```python
from build123d import *

# Parameters (mm, degrees)
BOSS_EXTRUDE1_DEPTH = 3
BOSS_EXTRUDE3_DEPTH = 0.5
SKETCH4_W           = 3
SKETCH4_H           = 0.5
BOSS_EXTRUDE5_DEPTH = 7.5
FILLET1_R           = 1.5


with BuildPart() as part:
    # Sketch1 → Boss-Extrude1 (new body)
    with BuildSketch(Plane.XY):
        with BuildLine():
            Line((0, 0), (1.5, 0))
            Line((1.5, 0), (7.55, -0.6))
            ThreePointArc((7.55, -0.6), (8, -1.05), (7.55, -1.5))
            Line((7.55, -1.5), (4.75, -1.5))
            Line((4.75, -1.5), (4.75, -7.5))
            Line((4.75, -7.5), (5.25, -7.5))
            Line((5.25, -7.5), (5.25, -2))
            Line((5.25, -2), (7.55, -2))
            ThreePointArc((7.55, -2), (8.5, -1.05), (7.55, -0.1))
            Line((7.55, -0.1), (1.5, 0.5))
            Line((1.5, 0.5), (0, 0.5))
            Line((0, 0.5), (0, 0))
        make_face()
    extrude(amount=BOSS_EXTRUDE1_DEPTH)

    # Sketch3 → Boss-Extrude3 (add)
    with BuildSketch(Plane(origin=(0, 0, 0), x_dir=(-1, 0, 0), z_dir=(0, -1, 0))):
        Polygon((-3, 1), (-1.5, 1), (-1.5, 0), (0, 0), (0, 3.5), (-3, 3.5), align=None)
    extrude(amount=-BOSS_EXTRUDE3_DEPTH)

    # Sketch4 → Boss-Extrude5 (add)
    with BuildSketch(Plane.XZ):
        with Locations((1.5, -3.25)):
            Rectangle(SKETCH4_W, SKETCH4_H)
    extrude(amount=BOSS_EXTRUDE5_DEPTH)

    # Fillet1
    fillet1_edges = [part.edges().sort_by_distance(p)[0] for p in [
        (0, -7.5, -3.25),
        (3, -7.5, -3.25),
        (5, -7.5, 3),
        (5, -7.5, 0),
    ]]
    fillet(fillet1_edges, radius=FILLET1_R - 0.0001)  # a hair under: the kernel refuses the full size


solid = part.part
```
Build history of the part. All positions in model axes, mm. A direction names the side the tool comes from. Round coordinates to 2 decimals unless told otherwise and drop trailing zeros. Loops run counter-clockwise (first coordinate to the right, second up) from the corner with the lowest first, then second, coordinate; pieces in that order, holes last. Notation, with made-up numbers: M 12,10.5 L 34,10.5 A22 cw 34,30.5 Z; hole C 48.5,70 d9. An arc over 180 degrees is marked long. Answer as CSV lines item,"result".
1. Flat gauge pins, fed straight in: P1, Ø2, axis at x = 3.5, y = -4.5, coming from the -Z side; P2, Ø3, axis at y = -3, z = -2, coming from the +X side; P3, Ø1, axis at y = -3, z = 0, coming from the +X side; P4, Ø1.2, axis at x = 6, z = 1.5, coming from the -Y side. Where does each tip first touch, or does it go through?
Resolved:
P1,"stops at z = -3.5"
P2,"stops at x = 3"
P3,"stops at x = 5.25"
P4,"stops at y = -2"
2. Two-plate mould, pull along Y, no slides. Class faces 5 (the flat face through (6, -1.5, 1)), 6 (the cylindrical face through (5, -7.05, 0.43)), 7 (the cylindrical face through (8.5, -1.1, 1.5)), 8 (the flat face through (0, -1.3, -3.2)): released by +Y, released by -Y, zero draft, split by the parting line, or undercut.
Resolved:
face 5,"undercut"
face 6,"released by -Y"
face 7,"split by the parting line"
face 8,"zero draft"
3. Wall check: probe 1 along Z at (x, y) = (1.75, -3.5); probe 2 along X at (y, z) = (-6, 2); probe 3 along Y at (x, z) = (5.75, 2.25). Give the ranges that are in metal, low to high. Write a range as [from, to].
Resolved:
probe 1,"z = [-3.5, -3]"
probe 2,"x = [4.75, 5.25]"
probe 3,"y = [-2, -1.5], [-0.42, 0.08]"
4. 3-axis set-ups, long thin cutter, end or side, ignore diameter. For faces 1 (the flat face through (4.483, -0.296, 1.479)), 2 (the flat face through (1, 0, -1)), 3 (the flat face through (4.75, -4, 1)), 4 (the flat face through (6, -2, 1)): which of +Z, -Z, +X, -X, +Y, -Y reach the whole face in a straight line?
Resolved:
face 1,"+Z, -X"
face 2,"-X, -Y"
face 3,"+Z, -Z, -X, -Y"
face 4,"+Z, -Z, +X, -Y"
5. Cut at C-C on x = 2.25. Write the cut outline in (y, z), then the cut area to 3 significant figures.
Resolved:
outline,"M -7.3,-3.5 L 0.5,-3.5 L 0.5,-1 L 0,-1 L 0,-3 L -7.3,-3 Z; M -0.07,0 L 0.43,0 L 0.43,3 L -0.07,3 Z"
area,"6.40 mm²"
6. Cut at A-A on y = -1.05. Write the cut outline in (x, z).
Resolved:
outline,"M 0,-3.5 L 3,-3.5 L 3,-3 L 0,-3 Z; M 8,0 L 8.5,0 L 8.5,3 L 8,3 Z"
7. Cut at D-D on z = -1.5. Write the cut outline in (x, y), then the cut area to 3 significant figures.
Resolved:
outline,"M 0,0 L 3,0 L 3,0.5 L 0,0.5 Z"
area,"1.50 mm²"
8. Cut at B-B on x = 7.25. Write the cut outline in (y, z).
Resolved:
outline,"M -2,0 L -1.5,0 L -1.5,3 L -2,3 Z; M -0.57,0 L -0.07,0 L -0.07,3 L -0.57,3 Z"
